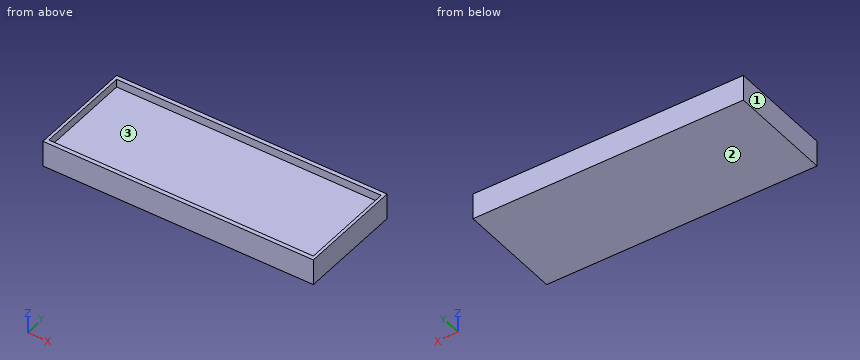
```python
from build123d import *

# Parameters (mm, degrees)
SKETCH002_W      = 323.85
SKETCH002_H      = 118.618
EXTRUDE002_DEPTH = 9.906
SKETCH001_W      = 323.85
SKETCH001_H      = 128.778
EXTRUDE001_DEPTH = 9.906
SKETCH_W         = 330.99375
SKETCH_H         = 128.778
EXTRUDE_DEPTH    = 31.75


with BuildPart() as extrude002:
    # Sketch002 (on Face6 of Cut) → Extrude002 (new body)
    with BuildSketch(Plane.XY.offset(31.75)):
        Rectangle(SKETCH002_W, SKETCH002_H)
    extrude(amount=-EXTRUDE002_DEPTH)


with BuildPart() as extrude001:
    # Sketch001 (on Face6 of Extrude) → Extrude001 (new body)
    with BuildSketch(Plane.XY.offset(31.75)):
        with Locations((334.565625, 0)):
            Rectangle(SKETCH001_W, SKETCH001_H)
    extrude(amount=-EXTRUDE001_DEPTH)


with BuildPart() as cut001:
    # Sketch → Extrude (new body)
    with BuildSketch(Plane.XY):
        Rectangle(SKETCH_W, SKETCH_H)
    extrude(amount=EXTRUDE_DEPTH)

    # Cut: cut Extrude001
    add(extrude001.part, mode=Mode.SUBTRACT)

    # Cut001: cut Extrude002
    add(extrude002.part, mode=Mode.SUBTRACT)


solid = cut001.part
```
CAD build for the part. Positions are in the model's coordinates, mm. Face numbers are marked on the shaded views. Round coordinates to 2 decimals unless told otherwise and drop trailing zeros. Order: outer loops, then holes, each group sorted by start corner. A loop starts at its lowest first (then second) coordinate and runs counter-clockwise, first axis right, second up. Notation, with made-up numbers: (48, 15.25) - (60, 15.25) arc R22 cw to (60, 52.25) - close; hole circle Ø11 at (76, -23). An arc over 180 degrees is marked (long way). Answer in a Markdown table with one row per item. Add a question column.
(1) Probe L1, parallel to X at y = -34, z = 30.5 (3 decimals); L2, parallel to Y at x = 152, z = 26; L3, parallel to Z at x = 58, y = 38.5. List the from-to ranges inside material, lowest first. Write a range as [from, to].
(2) Band-saw the part on C-C on y = 55. List the corners of the cut face in (x, z) (3 decimals), and give its area (3 significant figures).
(3) Mould opens along X. For the marked faces 1, 2 and 3 say: +X half, -X half, draft (parallel to the pull), parting line (faces both ways), or undercut.
(4) Band-saw the part on B-B on z = 26. List the corners of the cut face in (x, y) (3 decimals), and give its area (3 significant figures).
(5) Drop a flat-ended pin along its axis: pin 1 Ø6 at (x, y) = (-4.5, -10.5) entering from -Z. Give the stop position or say it passes through.
(6) Band-saw the part on A-A on x = -35. List the corners of the cut face in (y, z).
Data:
| question | item | result |
|---|---|---|
| 1 | L1 | x = [-165.497, -161.925], [161.925, 165.497] |
| 1 | L2 | y = [-64.39, -59.31], [59.31, 64.39] |
| 1 | L3 | z = [0, 21.84] |
| 2 | outline | (-165.497, 0) - (165.497, 0) - (165.497, 31.75) - (161.925, 31.75) - (161.925, 21.844) - (-161.925, 21.844) - (-161.925, 31.75) - (-165.497, 31.75) - close |
| 2 | area | 7,300 mm^2 |
| 3 | face 1 | -X half |
| 3 | face 2 | draft |
| 3 | face 3 | undercut |
| 4 | outline | (-165.497, -64.389) - (165.497, -64.389) - (165.497, 64.389) - (-165.497, 64.389) - close; hole (-161.925, -59.309) - (161.925, -59.309) - (161.925, 59.309) - (-161.925, 59.309) - close |
| 4 | area | 4,210 mm^2 |
| 5 | pin 1 | stops at z = 0 |
| 6 | outline | (-64.39, 0) - (64.39, 0) - (64.39, 31.75) - (59.31, 31.75) - (59.31, 21.84) - (-59.31, 21.84) - (-59.31, 31.75) - (-64.39, 31.75) - close |
